```python
from build123d import *

# Parameters (mm, degrees)
SKETCH1_W           = 35
SKETCH1_H           = 70
CUT_EXTRUDE17_DEPTH = 2.5
CUT_EXTRUDE25_DEPTH = 116


with BuildPart() as part:
    # Sketch1 → Revolve1 (revolve)
    with BuildSketch(Plane.XY, mode=Mode.PRIVATE) as revolve1_sk:
        with Locations((17.5, 35)):
            Rectangle(SKETCH1_W, SKETCH1_H)
    revolve(revolve1_sk.sketch.rotate(Axis((0, 0, 0), (0, 1, 0)), 90), axis=Axis((0, 0, 0), (0, 1, 0)))

    # 3DSketch2 → Cut-Extrude17 (cut)
    with BuildSketch(Plane(origin=(-32.691742077, 65, 12.5), x_dir=(0, -0.923076923076923, -0.38461538461538475), z_dir=(1, 0, 0))):
        Polygon((0, 0), (9.615384615, 23.076923077), (65, 0), (55.384615385, -23.076923077), align=None)
    extrude(amount=-CUT_EXTRUDE17_DEPTH, mode=Mode.SUBTRACT)

    # 3DSketch3 → Cut-Extrude25 (cut, along a direction that is not the sketch's normal)
    with BuildSketch(Plane(origin=(-18.666557597, 54.986311826, -29.606749695), x_dir=(0.6694273156469549, -0.7427399140993083, -0.014299967463753989), z_dir=(0.021356621715658074, -1.1658435530169433e-15, 0.9997719213445107))):
        Polygon((0, 0), (24.145055974, 26.783201302), (53.854652538, 0), (29.709596564, -26.783201302), align=None)
    extrude(amount=-CUT_EXTRUDE25_DEPTH, dir=(0, 0, 1), mode=Mode.SUBTRACT)


solid = part.part
```
Build history of the part. All positions in model axes, mm. A direction names the side the tool comes from. Give positions to 0.01 mm unless a question says otherwise; leave off trailing zeros. Loops run counter-clockwise (first coordinate to the right, second up) from the corner with the lowest first, then second, coordinate; pieces in that order, holes last.
Item 1: Slice it at D-D, the plane z = 21. List the corners of the cut face in (x, y), and give its area (3 significant figures).
Answers follow:
outline: (-28, 0) - (28, 0) - (28, 70) - (-28, 70) - close
area: 3,920 mm2
Item 2: Slice it at C-C, the plane x = -10. List the corners of the cut face in (y, z), and give its area (3 significant figures).
Answers follow:
outline: (0, -33.54) - (14.99, -33.54) - (14.99, -29.79) - (54.99, -29.79) - (54.99, -33.54) - (70, -33.54) - (70, 33.54) - (0, 33.54) - close
area: 4,550 mm2
Item 3: Pull direction Y, two halves, no side cores. Call faces 1 (the face through (0, 0, 0)), 2 (the face through (0, 70, 0)), 3 (the face through (-32.692, 35, 0)): released by +Y, released by -Y, zero draft, split by the parting line, or undercut.
Answers follow:
face 1: released by -Y
face 2: released by +Y
face 3: undercut
Item 4: Slice it at B-B, the plane y = 33. List the corners of the cut face in (x, z), and give its area (3 significant figures).
Answers follow:
outline: (-32.69, -12.5) arc R35 ccw to (-18.67, -29.61) - (17.39, -30.38) arc R35 ccw (long way) to (-32.69, 12.5) - close
area: 3,690 mm2
Item 5: Drill centre lines: line 1 (Y direction, x = -15, z = -31); line 2 (X direction, y = 37, z = 1); line 3 (Z direction, x = 8.5, y = 16). Where is each one in solid material? Low to high.
Answers follow:
line 1: y = 0 to 14.99, 54.99 to 70
line 2: x = -32.69 to 34.99
line 3: z = -30.19 to 33.95
Item 6: Slice it at A-A, the plane z = 0. List the corners of the cut face in (x, y), and give its area (3 significant figures).
Answers follow:
outline: (-35, 0) - (35, 0) - (35, 70) - (-35, 70) - (-35, 65) - (-32.69, 65) - (-32.69, 5) - (-35, 5) - close
area: 4,760 mm2
Item 7: Which spindle directions (+Z, -Z, +X, -X, +Y, -Y) get a long thin tool onto all of the face, cutting with end or side? Do faces 4 (the face through (21, 35, 28)), 5 (the face through (-34, 65, 0)). Say none if no direction does.
Answers follow:
face 4: +Y, -Y
face 5: +Z, -Z, -X
Item 8: Flat gauge pins, fed straight in: pin 1 (1.6 mm diameter, centred on x = 4.5, z = -33, fed in from -Y); pin 2 (8 mm diameter, centred on y = 52.5, z = -2, fed in from +X); pin 3 (8 mm diameter, centred on x = 27, y = 30.5, fed in from -Z). Where does each tip first touch, or does it go through?
Answers follow:
pin 1: stops at y = 0
pin 2: stops at x = 35
pin 3: stops at z = -26.38
